Here's how the part is built. I have some questions about the finished solid (model axes, mm). A direction names the side the tool comes from. Give positions to 0.01 mm unless a question says otherwise; leave off trailing zeros. Write each loop counter-clockwise with the first axis right and the second up, starting at its lowest first coordinate (ties: lowest second). Pieces come first, ordered by that corner, then holes. Notation, with made-up numbers: M -5.75,23.25 L 23.25,23.25 A11 ccw 23.25,39.25 Z; hole C -11,68 d1. An arc over 180 degrees is marked long. Answer as CSV lines item,"result". Start each with the question number.
Q1. If I drill on line 1 along Y through (x, z) = (0, 2.85); line 2 along Y through (x, z) = (1.5, 1.7); line 3 along X through (y, z) = (-10.5, 3.3), over which ranges is the centre line in solid material (lowest first)?
Q2. On a 3-axis mill with a long thin cutter (end or side, diameter ignored), from which of +Z, -Z, +X, -X, +Y, -Y can I reach the whole of each face in a straight line? I mean faces 5 (the cylindrical face through (-0.21, -12.31, 2.46)), 6 (the cylindrical face through (1.844, 14.886, 2.465)), 7 (the flat face through (-15, -8.592, 2)). Say none if no direction works.
Q3. Suppose I cut it at C-C (z = 1.3). Count the separate pieces of the cut face and the enclosed holes in it, then the cut area to 3 significant figures.
Q4. For pin 1 (0.6 mm diameter, centred on x = 15, z = 3.5, fed in from -Y); pin 2 (3 mm diameter, centred on x = -2, z = 2, fed in from +Y); pin 3 (2.5 mm diameter, centred on x = -5.51, y = 7.55, fed in from +Z); pin 4 (3 mm diameter, centred on x = 5, z = 1.5, fed in from +Y), each with a flat end and sliding along its axis, tell me the tip position at first contact or that it passes through.
Q5. Thinking about a two-plate mould opening in X: for faces 1 (the flat face through (-1, -3, 5)), 2 (the cylindrical face through (-4.567, 5.725, 2.465)), 3 (the flat face through (-2.31, 18.07, 2.46)), 4 (the flat face through (-5.488, 17.471, 2.465)), which applies, +X half, -X half, draft (parallel to the pull), parting line (faces both ways), or undercut?
Q6. Suppose I cut it at B-B (y = 6). Write out the boundary of the cut face in (x, z).
Q7. Suppose I cut it at A-A (y = 0). Write out the boundary of the cut face in (x, z).
Q8. Suppose I cut it at D-D (x = -11.5). Write out the boundary of the cut face in (y, z), then the cut area to 3 significant figures.
```python
from build123d import *

# Parameters (mm, degrees)
F0_R     = 1.9348900532
F0_R_2   = 2.0522604458
F0_R_3   = 2.3419360145
F1_DEPTH = 5


with BuildPart() as f1:
    # F0 (on Top) → F1 (new body)
    with BuildSketch(Plane.XY):
        with BuildLine():
            Line((14.5436545132, -3.6717997494), (14.5436545132, 3.6717997494))
            ThreePointArc((14.5436545132, 3.6717997494), (12.5272279605, 8.2503672419), (9.117258298, 11.9111544834))
            ThreePointArc((9.117258298, 11.9111544834), (6.4998434958, 13.5185810842), (3.6098778188, 14.5591477132))
            ThreePointArc((3.6098778188, 14.5591477132), (1.818348743, 14.8893790283), (0, 15))
            ThreePointArc((0, 15), (-3.2325615836, 14.6475440129), (-6.3132117426, 13.6067394145))
            ThreePointArc((-6.3132117426, 13.6067394145), (-11.7007085883, 9.3858094234), (-14.6523065602, 3.2109052408))
            Line((-14.6523065602, 3.2109052408), (-13.6017017066, 3.2109052408))
            Line((-13.6017017066, 3.2109052408), (-13.6017017066, -6.3240580867))
            ThreePointArc((-13.6017017066, -6.3240580867), (-11.0937814491, -10.0959404297), (-7.5742680527, -12.9472183679))
            ThreePointArc((-7.5742680527, -12.9472183679), (-5.5179001004, -13.0164836252), (-4.0382475823, -14.4461952245))
            ThreePointArc((-4.0382475823, -14.4461952245), (-1.3916396268, -14.9353051241), (1.2997714686, -14.9435803651))
            ThreePointArc((1.2997714686, -14.9435803651), (3.4559828028, -13.1380275344), (6.2215345161, -13.6489013574))
            ThreePointArc((6.2215345161, -13.6489013574), (11.5188501154, -9.6081263532), (14.5436545132, -3.6717997494))
        make_face()
        with BuildLine():
            ThreePointArc((5.7079247199, -6.2883910723), (-0.3391810804, -12.3095638451), (-6.2883906066, -6.1916462146))
            Line((-6.2883906066, -6.1916462146), (-4.8886678044, -6.2194979452))
            ThreePointArc((-4.8886678044, -6.2194979452), (-0.3278910818, -10.9096094966), (4.3079347792, -6.2936643859))
            Line((4.3079347792, -6.2936643859), (5.7079247199, -6.2883910723))
        make_face(mode=Mode.SUBTRACT)
        Circle(F0_R, mode=Mode.SUBTRACT)
        with Locations((-5.5144345388, 7.5460691005)):
            Circle(F0_R_2, mode=Mode.SUBTRACT)
        with Locations((5.0307135098, 7.1590915322)):
            Circle(F0_R_3, mode=Mode.SUBTRACT)
        with BuildLine():
            ThreePointArc((1.2997714686, -14.9435803651), (3.8159611322, -14.5064964977), (6.2215345161, -13.6489013574))
            ThreePointArc((6.2215345161, -13.6489013574), (3.4559828028, -13.1380275344), (1.2997714686, -14.9435803651))
        make_face()
        with BuildLine():
            ThreePointArc((7.5981171759, -16.3314789534), (7.2338832803, -14.8238979126), (6.2215345161, -13.6489013574))
            ThreePointArc((6.2215345161, -13.6489013574), (3.8159611322, -14.5064964977), (1.2997714686, -14.9435803651))
            ThreePointArc((1.2997714686, -14.9435803651), (3.5854281507, -19.5562045673), (7.5981171759, -16.3314789534))
        make_face()
        with BuildLine():
            ThreePointArc((-3.7710910204, -15.6542677432), (-3.8386773507, -15.0356378379), (-4.0382475823, -14.4461952245))
            ThreePointArc((-4.0382475823, -14.4461952245), (-5.8544310354, -13.8103452981), (-7.5742680527, -12.9472183679))
            ThreePointArc((-7.5742680527, -12.9472183679), (-8.297487219, -17.9883774161), (-3.7710910204, -15.6542677432))
        make_face()
        with BuildLine():
            ThreePointArc((-7.5742680527, -12.9472183679), (-5.8544310354, -13.8103452981), (-4.0382475823, -14.4461952245))
            ThreePointArc((-4.0382475823, -14.4461952245), (-5.5179001004, -13.0164836252), (-7.5742680527, -12.9472183679))
        make_face()
        with BuildLine():
            ThreePointArc((14.5436545132, 3.6717997494), (14.8854764401, 1.8500246352), (15, 0))
            ThreePointArc((15, 0), (14.8854764401, -1.8500246352), (14.5436545132, -3.6717997494))
            Line((14.5436545132, -3.6717997494), (14.5436545132, -8.978898637))
            Line((14.5436545132, -8.978898637), (15.3239746839, -8.978898637))
            ThreePointArc((15.3239746839, -8.978898637), (16.7381882463, -8.3931121994), (17.3239746839, -6.978898637))
            Line((17.3239746839, -6.978898637), (17.3239746839, 1.6717997494))
            ThreePointArc((17.3239746839, 1.6717997494), (16.7381882463, 3.0860133118), (15.3239746839, 3.6717997494))
            Line((15.3239746839, 3.6717997494), (14.5436545132, 3.6717997494))
        make_face()
        with BuildLine():
            ThreePointArc((14.5436545132, -3.6717997494), (14.8854764401, -1.8500246352), (15, 0))
            ThreePointArc((15, 0), (14.8854764401, 1.8500246352), (14.5436545132, 3.6717997494))
            Line((14.5436545132, 3.6717997494), (14.5436545132, -3.6717997494))
        make_face()
        with BuildLine():
            ThreePointArc((-13.6017017066, -6.3240580867), (-14.9097661685, -1.6428246406), (-14.6523065602, 3.2109052408))
            Line((-14.6523065602, 3.2109052408), (-16.4389259666, 3.2109052408))
            ThreePointArc((-16.4389259666, 3.2109052408), (-17.853139529, 2.6251188032), (-18.4389259666, 1.2109052408))
            Line((-18.4389259666, 1.2109052408), (-18.4389259666, -6.5919210687))
            ThreePointArc((-18.4389259666, -6.5919210687), (-17.853139529, -8.0061346311), (-16.4389259666, -8.5919210687))
            Line((-16.4389259666, -8.5919210687), (-13.6017017066, -8.5919210687))
            Line((-13.6017017066, -8.5919210687), (-13.6017017066, -6.3240580867))
        make_face()
        with BuildLine():
            Line((-13.6017017066, 3.2109052408), (-14.6523065602, 3.2109052408))
            ThreePointArc((-14.6523065602, 3.2109052408), (-14.9097661685, -1.6428246406), (-13.6017017066, -6.3240580867))
            Line((-13.6017017066, -6.3240580867), (-13.6017017066, 3.2109052408))
        make_face()
        with BuildLine():
            ThreePointArc((-6.3132117426, 13.6067394145), (-3.2325615836, 14.6475440129), (0, 15))
            Line((0, 15), (-4.6849409118, 21.2286375463))
            Line((-4.6849409118, 21.2286375463), (-6.3132117426, 13.6067394145))
        make_face()
        with BuildLine():
            ThreePointArc((3.6098778188, 14.5591477132), (6.4998434958, 13.5185810842), (9.117258298, 11.9111544834))
            Line((9.117258298, 11.9111544834), (6.734602619, 21.0822317749))
            Line((6.734602619, 21.0822317749), (3.6098778188, 14.5591477132))
        make_face()
    extrude(amount=F1_DEPTH)


solid = f1.part
```
Resolved:
1,line 1,"-15 to -12.3, -10.9 to -1.93, 1.93 to 15"
1,line 2,"-18.09 to -12.04, -10.55 to -1.22, 1.22 to 14.92"
1,line 3,"-10.71 to -4.58, -2.19 to 1.61, 4 to 10.71"
2,face 5,"+Z, -Z"
2,face 6,"+Z, -Z, +Y"
2,face 7,"+Z, -Z, -X, -Y"
3,separate pieces,"1"
3,enclosed holes,"4"
3,area,"813 mm^2"
4,pin 1,"y = -8.98"
4,pin 2,"y = 19.65"
4,pin 3,"through"
4,pin 4,"y = 20.59"
5,face 1,"draft"
5,face 2,"undercut"
5,face 3,"undercut"
5,face 4,"-X half"
6,outline,"M -13.75,0 L -6.86,0 L -6.86,5 L -13.75,5 Z; M -4.16,0 L 3,0 L 3,5 L -4.16,5 Z; M 7.07,0 L 13.75,0 L 13.75,5 L 7.07,5 Z"
7,outline,"M -18.44,0 L -1.93,0 L -1.93,5 L -18.44,5 Z; M 1.93,0 L 17.32,0 L 17.32,5 L 1.93,5 Z"
8,outline,"M -9.63,0 L 9.63,0 L 9.63,5 L -9.63,5 Z"
8,area,"96.3 mm^2"
